Drawing for the job (mm, zero at the part's lowest x, y, z). A direction names the side the tool comes from. Coordinates: 2 decimals unless noted, no trailing zeros. Order: outer loops, then holes, each group sorted by start corner. A loop starts at its lowest first (then second) coordinate and runs counter-clockwise, first axis right, second up. Notation, with made-up numbers: (30.25, 49) -> (59.25, 49) arc R11 ccw to (59.25, 57) -> close; hole circle Ø7 at (69, 30). An arc over 180 degrees is marked (long way). Write each question's results on one line, items separated by ' | '.
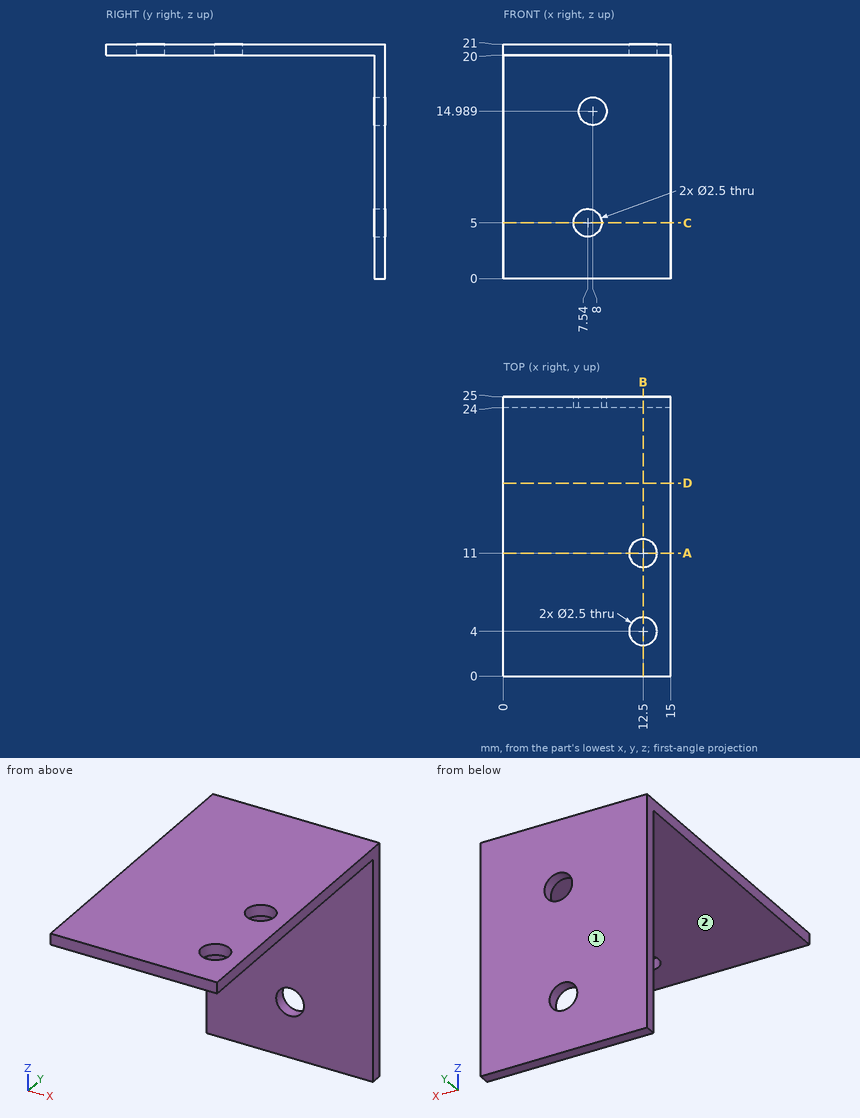
Item 1: Slice it at C-C, the plane z = 5. List the corners of the cut face in (x, y).
Answer:
outline: (0, 24) -> (6.29, 24) -> (6.29, 25) -> (0, 25) -> close; (8.79, 24) -> (15, 24) -> (15, 25) -> (8.79, 25) -> close
Item 2: Slice it at D-D, the plane y = 17.25. List the corners of the cut face in (x, z), and give its area (3 significant figures).
Answer:
outline: (0, 20) -> (15, 20) -> (15, 21) -> (0, 21) -> close | area: 15.0 mm^2
Item 3: Tool access for the marked faces 1 and 2: list every direction of +Z, -Z, +X, -X, +Y, -Y with a clear straight run to the whole face (end or side of a thin tool).
Answer:
face 1: +Z, -Z, +X, -X, +Y | face 2: -Z, +X, -X, -Y
Item 4: Slice it at A-A, the plane y = 11. List the corners of the cut face in (x, z).
Answer:
outline: (0, 20) -> (11.25, 20) -> (11.25, 21) -> (0, 21) -> close; (13.75, 20) -> (15, 20) -> (15, 21) -> (13.75, 21) -> close
Item 5: Drill centre lines: line 1 (Y direction, x = 12.5, z = 20.65); line 2 (X direction, y = 24.45, z = 5); line 3 (Y direction, x = 4.25, z = 11.25). Where is each one in solid material? Low to high. Write a range as from..to.
Answer:
line 1: y = 0..2.75, 5.25..9.75, 12.25..25 | line 2: x = 0..6.29, 8.79..15 | line 3: y = 24..25
Item 6: Pin check, flat tips, straight feed: pin 1 (1.5 mm diameter, centred on x = 1.5, y = 6.5, fed in from -Z); pin 2 (3 mm diameter, centred on x = 7.54, z = 5, fed in from -Y). Stop position of each tip, or through.
Answer:
pin 1: stops at z = 20 | pin 2: stops at y = 24
Item 7: Slice it at B-B, the plane x = 12.5. List the corners of the cut face in (y, z).
Answer:
outline: (0, 20) -> (2.75, 20) -> (2.75, 21) -> (0, 21) -> close; (5.25, 20) -> (9.75, 20) -> (9.75, 21) -> (5.25, 21) -> close; (12.25, 20) -> (24, 20) -> (24, 0) -> (25, 0) -> (25, 21) -> (12.25, 21) -> close
